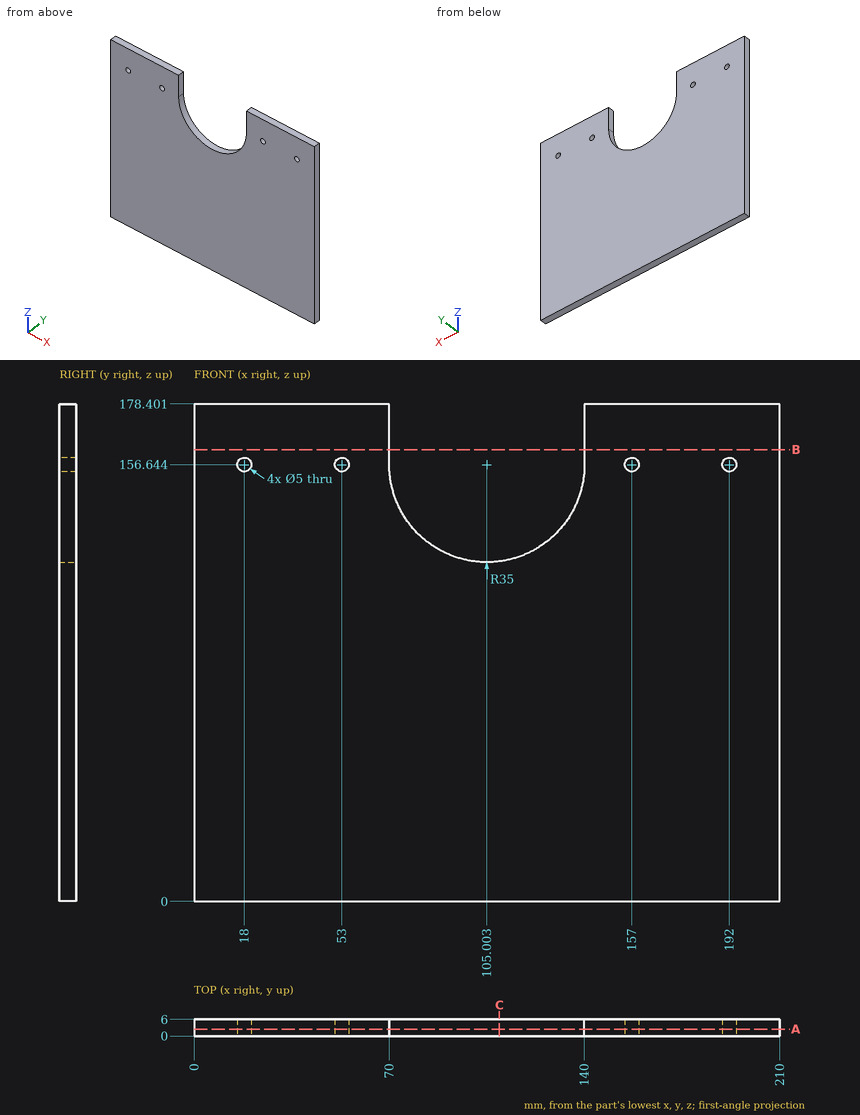
Could you check a few things on this drawing? It's one solid part, dimensions in mm from its lowest x, y, z. Round coordinates to 2 decimals unless told otherwise and drop trailing zeros. Loops run counter-clockwise (first coordinate to the right, second up) from the corner with the lowest first, then second, coordinate; pieces in that order, holes last. Notation, with made-up numbers: (39.25, 31.5) -> (60.25, 31.5) arc R5 cw to (60.25, 35.5) -> close; hole circle Ø3 at (-16, -39.5). An arc over 180 degrees is marked (long way). Write each question's results on one line, items separated by ' | '.
(1) If we section it at B-B, the plane z = 162: List the corners of the cut face in (x, y) for me.
Worked answers:
outline: (0, 0) -> (70, 0) -> (70, 6) -> (0, 6) -> close; (140, 0) -> (210, 0) -> (210, 6) -> (140, 6) -> close
(2) For P1, Ø6, axis at x = 192, z = 156.64, coming from the +Y side, with a flat end and sliding along its axis, tell me the tip position at first contact or that it passes through.
Worked answers:
P1: y = 6
(3) If we section it at C-C, the plane x = 109.5: List the corners of the cut face in (y, z) for me.
Worked answers:
outline: (0, 0) -> (6, 0) -> (6, 121.93) -> (0, 121.93) -> close
(4) If I drill on L1, parallel to X at y = 4.25, z = 168.5; L2, parallel to Z at x = 106.5, y = 4.55; L3, parallel to Z at x = 55, y = 4.2 (1 decimal), over which ranges is the centre line in solid material (lowest first)?
Worked answers:
L1: 0 to 70, 140 to 210 | L2: 0 to 121.68 | L3: 0 to 155.1, 158.1 to 178.4
(5) If we section it at A-A, the plane y = 2.45: List the corners of the cut face in (x, z) for me.
Worked answers:
outline: (0, 0) -> (210, 0) -> (210, 178.4) -> (140, 178.4) -> (140, 156.64) arc R35 cw to (70, 156.64) -> (70, 178.4) -> (0, 178.4) -> close; hole circle Ø5 at (18, 156.64); hole circle Ø5 at (53, 156.64); hole circle Ø5 at (157, 156.64); hole circle Ø5 at (192, 156.64)
